Autodesk Inventor part; units mm, degrees
ref_plane "YZ Plane" through (0, 0, 0) normal (1, 0, 0) x (0, 1, 0)
ref_plane "XZ Plane" through (0, 0, 0) normal (0, 1, 0) x (-1, 0, 0)
ref_plane "XY Plane" through (0, 0, 0) normal (0, 0, 1) x (1, 0, 0)
sketch "スケッチ1" plane through (0, 0, 0) normal (0, 1, 0) x (-1, 0, 0)
  circle A0 centre (0, 0) radius 4
  circle A1 centre (0, 0) radius 6
  dimension "d0" = 8
  dimension "d1" = 12
extrude "押し出し1" add sketch "スケッチ1" along normal blind 3.5
sketch "スケッチ2" plane through (0, 3.5, 0) normal (0, 1, 0) x (1, 0, 0)
  circle A0 centre (0, 0) radius 6
  circle A1 centre (0, 0) radius 6.8
  circle A2 centre (0, 0) radius 6
  dimension "d4" = 13.6
extrude "押し出し2" add sketch "スケッチ2" against normal blind 0.8
sketch "スケッチ3" plane through (0, 3.5, 0) normal (0, 1, 0) x (1, 0, 0)
  circle A0 centre (0, 0) radius 4
  circle A1 centre (0, 0) radius 4.5
  circle A2 centre (0, 0) radius 5.5
  dimension "d7" = 9
  dimension "d8" = 11
extrude "押し出し3" cut sketch "スケッチ3" against normal blind 0.3 contours A2
sketch "スケッチ4" plane through (0, 0, 0) normal (0, -1, 0) x (1, 0, 0)
  circle A0 centre (0, 0) radius 4
  circle A1 centre (0, 0) radius 4.5
  circle A2 centre (0, 0) radius 5.5
  dimension "d11" = 9
  dimension "d12" = 11
extrude "押し出し4" cut sketch "スケッチ4" against normal blind 0.3 contours A2
properties part number "Bearing_MF128ZZ" material "ステンレス鋼"
Input: part model. Units: mm. Frame: model coordinates. A direction names the side the tool comes from. Coordinates: 2 decimals unless noted, no trailing zeros. Loops run counter-clockwise (first coordinate to the right, second up) from the corner with the lowest first, then second, coordinate; pieces in that order, holes last. Notation, with made-up numbers: (62, 52) -> (72, 52) arc R15 cw to (72, 64) -> close; hole circle Ø9 at (23, -34). An arc over 180 degrees is marked (long way). Use a Markdown table: item, result.
1) Access query for faces 4 (the flat face through (3, 3.5, -3)), 5 (the flat face through (-5, 3.2, 0)). Directions: +Z, -Z, +X, -X, +Y, -Y. A direction counts if a zero-diameter tool reaches every point of the face in a straight line with its end or side. Return the directions, or none.
Results found:
| item | result |
|---|---|
| face 4 | +Z, -Z, +X, -X, +Y |
| face 5 | +Y |
2) Cut plane C-C (y = 1.8). Return the cut outline in (x, z), then the cut area to 3 significant figures.
Results found:
| item | result |
|---|---|
| outline | circle Ø12 at (0, 0); hole circle Ø8 at (0, 0) |
| area | 62.8 mm2 |
3) Material intervals for line 1 along Z through (x, y) = (0, 0.1); line 2 along Z through (x, y) = (0, 3.3); line 3 along Z through (x, y) = (0, 1.2), sorted ascending. Write a range as from..to.
Results found:
| item | result |
|---|---|
| line 1 | z = -6..-5.5, -4.5..-4, 4..4.5, 5.5..6 |
| line 2 | z = -6.8..-5.5, -4.5..-4, 4..4.5, 5.5..6.8 |
| line 3 | z = -6..-4, 4..6 |
4) Contact query for flat-ended pins moving along their axis: pin 1 (2 mm diameter, centred on x = 0, z = -5, fed in from +Y); pin 2 (2 mm diameter, centred on x = 4, y = 1.5, fed in from -Z); pin 3 (1 mm diameter, centred on x = 4, y = 1.5, fed in from +Z). Output: stop coordinate, or through.
Results found:
| item | result |
|---|---|
| pin 1 | stops at y = 3.5 |
| pin 2 | stops at z = -5.2 |
| pin 3 | stops at z = 4.87 |
5) Cut plane B-B (x = 0). Return the cut outline in (y, z).
Results found:
| item | result |
|---|---|
| outline | (0, -6) -> (2.7, -6) -> (2.7, -6.8) -> (3.5, -6.8) -> (3.5, -5.5) -> (3.2, -5.5) -> (3.2, -4.5) -> (3.5, -4.5) -> (3.5, -4) -> (0, -4) -> (0, -4.5) -> (0.3, -4.5) -> (0.3, -5.5) -> (0, -5.5) -> close; (0, 4) -> (3.5, 4) -> (3.5, 4.5) -> (3.2, 4.5) -> (3.2, 5.5) -> (3.5, 5.5) -> (3.5, 6.8) -> (2.7, 6.8) -> (2.7, 6) -> (0, 6) -> (0, 5.5) -> (0.3, 5.5) -> (0.3, 4.5) -> (0, 4.5) -> close |
6) Pull-direction query (Z, two-part tool) for faces 1 (the flat face through (-5, 0.3, 0)), 2 (the flat face through (4, 2.7, 5)), 3 (the cylindrical face through (6, 1, 0)); classes: released by +Z, released by -Z, zero draft, split by the parting line, or undercut.
Results found:
| item | result |
|---|---|
| face 1 | undercut |
| face 2 | zero draft |
| face 3 | split by the parting line |
7) Cut plane D-D (x = 5.25). Return the cut outline in (y, z), then the cut area to 3 significant figures.
Results found:
| item | result |
|---|---|
| outline | (0, -2.9) -> (2.7, -2.9) -> (2.7, -4.32) -> (3.5, -4.32) -> (3.5, -1.64) -> (3.2, -1.64) -> (3.2, 1.64) -> (3.5, 1.64) -> (3.5, 4.32) -> (2.7, 4.32) -> (2.7, 2.9) -> (0, 2.9) -> (0, 1.64) -> (0.3, 1.64) -> (0.3, -1.64) -> (0, -1.64) -> close |
| area | 20.6 mm2 |
8) Cut plane A-A (z = 0). Return the cut outline in (x, y), then the cut area to 3 significant figures.
Results found:
| item | result |
|---|---|
| outline | (-6.8, 2.7) -> (-6, 2.7) -> (-6, 0) -> (-5.5, 0) -> (-5.5, 0.3) -> (-4.5, 0.3) -> (-4.5, 0) -> (-4, 0) -> (-4, 3.5) -> (-4.5, 3.5) -> (-4.5, 3.2) -> (-5.5, 3.2) -> (-5.5, 3.5) -> (-6.8, 3.5) -> close; (4, 0) -> (4.5, 0) -> (4.5, 0.3) -> (5.5, 0.3) -> (5.5, 0) -> (6, 0) -> (6, 2.7) -> (6.8, 2.7) -> (6.8, 3.5) -> (5.5, 3.5) -> (5.5, 3.2) -> (4.5, 3.2) -> (4.5, 3.5) -> (4, 3.5) -> close |
| area | 14.1 mm2 |
